For this review, use the dimensioned drawing (mm, ordinates from the lowest corner) and the shaded views. Give positions to 0.01 mm unless a question says otherwise; leave off trailing zeros. Write each loop counter-clockwise with the first axis right and the second up, starting at its lowest first coordinate (ties: lowest second). Pieces come first, ordered by that corner, then holes. Notation, with made-up numbers: (52.25, 39) - (105.25, 39) arc R27 ccw to (105.25, 74) - close; hole circle Ø7 at (86.25, 46). An arc over 180 degrees is marked (long way). Use a Markdown table: item, result. Add a question column.
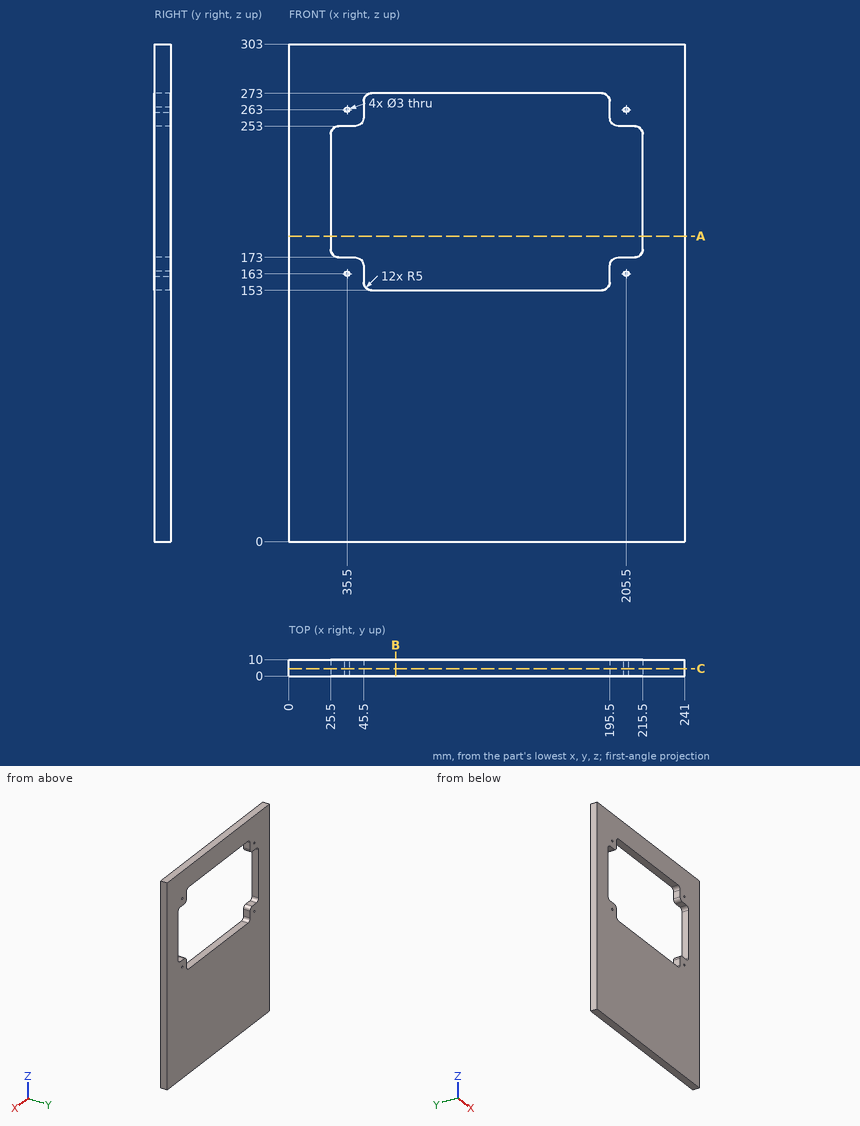
(1) Insertion check: pin 1 (2.5 mm diameter, centred on x = 35.5, z = 263, fed in from +Y). The pin has a flat end and moves straight along its axis. Give the tip position at first contact, or say it passes through.
(2) Add section A-A (z = 186). State the section outline as (x, y) points.
(3) Add section B-B (x = 65). State the section outline as (y, z) points, and give its area (3 significant figures).
(4) Add section C-C (y = 4.5). Count the separate pieces of the cut face and the enclosed holes in it, and give its area (3 significant figures).
(5) For line 1 along Z through (x, y) = (205.5, 6); line 2 along X through (y, z) = (6.25, 163); line 3 along Z through (x, y) = (190, 1.5), list the stretches that pass through material, from the lowest coordinate up.
Answers follow:
| question | item | result |
|---|---|---|
| 1 | pin 1 | through |
| 2 | outline | (0, 0) - (25.5, 0) - (25.5, 10) - (0, 10) - close; (215.5, 0) - (241, 0) - (241, 10) - (215.5, 10) - close |
| 3 | outline | (0, 0) - (10, 0) - (10, 153) - (0, 153) - close; (0, 273) - (10, 273) - (10, 303) - (0, 303) - close |
| 3 | area | 1,830 mm^2 |
| 4 | separate pieces | 1 |
| 4 | enclosed holes | 5 |
| 4 | area | 51,800 mm^2 |
| 5 | line 1 | 0 to 161.5, 164.5 to 173, 253 to 261.5, 264.5 to 303 |
| 5 | line 2 | 0 to 34, 37 to 45.5, 195.5 to 204, 207 to 241 |
| 5 | line 3 | 0 to 153, 273 to 303 |
